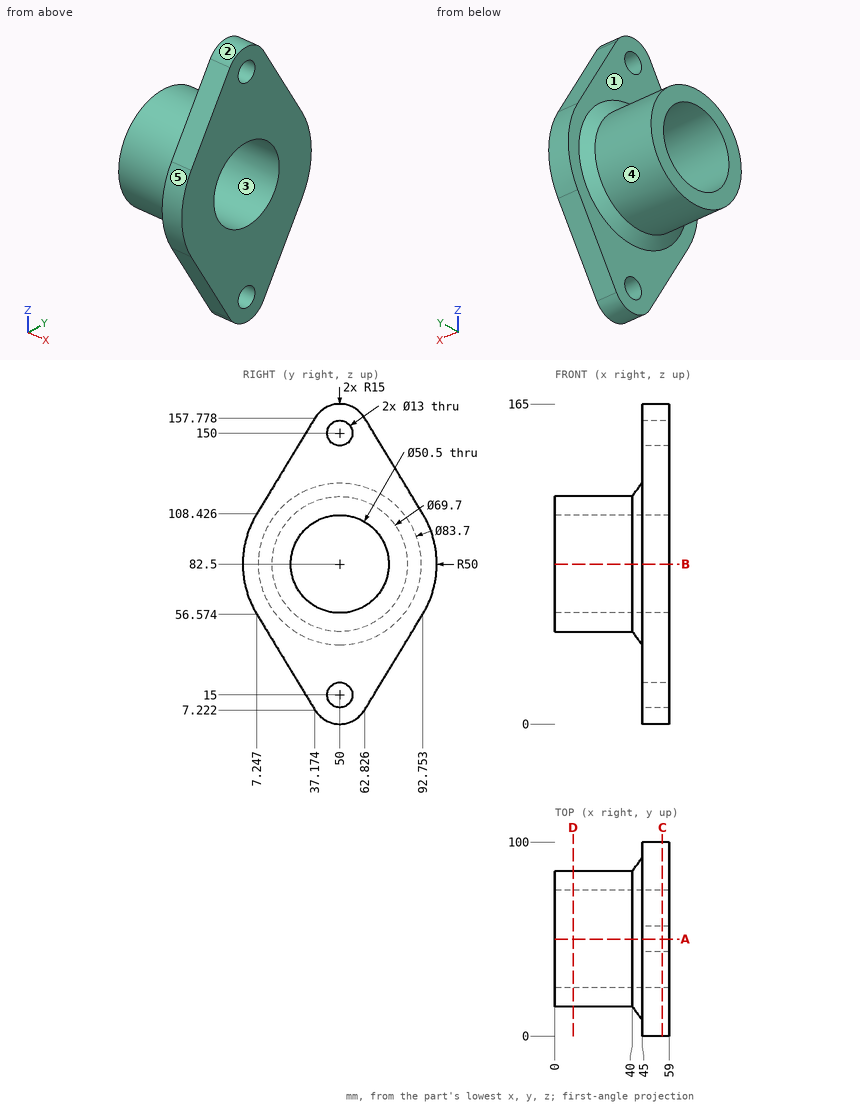
Design review of the part shown in the three views and the two pictorial views. Dimensions are in mm from the part's minimum x, y and z. A direction names the side the tool comes from. Round coordinates to 2 decimals unless told otherwise and drop trailing zeros. Write each loop counter-clockwise with the first axis right and the second up, starting at its lowest first coordinate (ties: lowest second). Pieces come first, ordered by that corner, then holes.
Item 1: For probe 1 along Y at (x, z) = (14, 82.5); probe 2 along Z at (x, y) = (7, 67.5); probe 3 along Z at (x, y) = (6, 68), list the stretches that pass through material, from the lowest coordinate up.
Item 2: We need section D-D on x = 9.5. Write out the cut boundary in (y, z).
Item 3: We need section C-C on x = 55.5. Write out the cut boundary in (y, z), and give its area (3 significant figures).
Item 4: We need section A-A on y = 50. Write out the cut boundary in (x, z).
Item 5: Clearance check with flat-ended pins moving along their axes: pin 1 Ø8 at (x, z) = (38.5, 98) entering from -Y; pin 2 Ø5 at (y, z) = (71.5, 148) entering from -X; pin 3 Ø1.5 at (x, y) = (19.5, 41.5) entering from +Z; pin 4 Ø17 at (y, z) = (50, 15) entering from +X. State where each tip first meets the part, or that it passes through.
Item 6: For the marked faces 4 and 5, list the 3-axis set-ups (+Z, -Z, +X, -X, +Y, -Y) from which the entire face can be reached by the end or side of a thin tool; tool diameter is ignored.
Item 7: We need section B-B on z = 82.5. Write out the cut boundary in (x, y).
Item 8: The part is to be moulded in two halves that separate along Y. For the marked faces 1, 2 and 3, say which applies: +Y half, -Y half, draft (parallel to the pull), parting line (faces both ways), or undercut.
Returned:
1. probe 1: y = 15.15 to 24.75, 75.25 to 84.85
1. probe 2: z = 52.36 to 64.3, 100.7 to 112.64
1. probe 3: z = 52.66 to 64.79, 100.21 to 112.34
2. outline: circle Ø69.7 at (50, 82.5); hole circle Ø50.5 at (50, 82.5)
3. outline: (7.25, 56.57) - (37.17, 7.22) arc R15 ccw to (62.83, 7.22) - (92.75, 56.57) arc R50 ccw to (92.75, 108.43) - (62.83, 157.78) arc R15 ccw to (37.17, 157.78) - (7.25, 108.43) arc R50 ccw to start; hole circle Ø50.5 at (50, 82.5); hole circle Ø13 at (50, 15); hole circle Ø13 at (50, 150)
3. area: 8,420 mm2
4. outline: (0, 47.65) - (40, 47.65) - (45, 40.65) - (45, 21.5) - (59, 21.5) - (59, 57.25) - (0, 57.25) - close; (0, 107.75) - (59, 107.75) - (59, 143.5) - (45, 143.5) - (45, 124.35) - (40, 117.35) - (0, 117.35) - close; (45, 0) - (59, 0) - (59, 8.5) - (45, 8.5) - close; (45, 156.5) - (59, 156.5) - (59, 165) - (45, 165) - close
5. pin 1: stops at y = 14.69
5. pin 2: stops at x = 45
5. pin 3: stops at z = 116.48
5. pin 4: stops at x = 59
6. face 4: -X
6. face 5: +X, -X, -Y
7. outline: (0, 15.15) - (40, 15.15) - (45, 8.15) - (45, 0) - (59, 0) - (59, 24.75) - (0, 24.75) - close; (0, 75.25) - (59, 75.25) - (59, 100) - (45, 100) - (45, 91.85) - (40, 84.85) - (0, 84.85) - close
8. face 1: draft
8. face 2: parting line
8. face 3: undercut
